```python
from build123d import *

# Parameters (mm, degrees)
TABAN_FLAN_1_DEPTH     = 5
IZGIDEN_START          = -60
IZGIDEN_B_KME2_DEPTH   = 60
IZGIDEN_B_KME2_2_DEPTH = 60
IZIM8_R                = 4.25
KES_EKSTR_ZYON1_DEPTH  = 10
RADYUS1_R              = 20
RADYUS2_R              = 5
IZIM9_R                = 4.25
KES_EKSTR_ZYON2_DEPTH  = 19


# Read off the part's stored shape, not the designer's step: Çizgiden Bükme2
# Sheet-metal steps are written as plain solids
with BuildPart() as part:
    # Çizim1 → Taban-Flanş1 (new body)
    with BuildSketch(Plane.XY):
        Polygon((0, 0), (-80, 0), (-120, -60), (-120, -115), (-50, -115), (-50, -60), (0, -60), align=None)
    extrude(amount=-TABAN_FLAN_1_DEPTH)

    # Çizgiden Bükme2 outline → Çizgiden Bükme2 (cut)
    with BuildSketch(Plane(origin=(0, 0, 0), x_dir=(1, 0, 0), z_dir=(0, 1, 0)).offset(IZGIDEN_START)):
        with BuildLine():
            Line((0, 5), (-31.042830313, 5))
            ThreePointArc((-31.042830313, 5), (-34.361671571, 1.351470729), (-39.105088062, 0))
            Line((-39.105088062, 0), (0, 0))
            Line((0, 0), (0, 5))
        make_face()
    extrude(amount=IZGIDEN_B_KME2_DEPTH, mode=Mode.SUBTRACT)

    # izgiden B_kme2 2 outline → izgiden B_kme2 2 (add)
    with BuildSketch(Plane(origin=(0, 0, 0), x_dir=(1, 0, 0), z_dir=(0, 1, 0)).offset(IZGIDEN_START)):
        with BuildLine():
            Line((-30.105088062, 37.894911938), (-35.105088062, 37.894911938))
            Line((-35.105088062, 37.894911938), (-35.105088062, 9))
            ThreePointArc((-35.105088062, 9), (-36.276660937, 6.171572875), (-39.105088062, 5))
            Line((-39.105088062, 5), (-31.042830313, 5))
            ThreePointArc((-31.042830313, 5), (-30.342659182, 6.945775053), (-30.105088062, 9))
            Line((-30.105088062, 9), (-30.105088062, 37.894911938))
        make_face()
    extrude(amount=IZGIDEN_B_KME2_2_DEPTH)

    # Çizim8 → Kes-Ekstrüzyon1 (cut)
    with BuildSketch(Plane.XY):
        with Locations((-70, -90)):
            Circle(IZIM8_R)
        with Locations((-95, -90)):
            Circle(IZIM8_R)
    extrude(amount=-KES_EKSTR_ZYON1_DEPTH, mode=Mode.SUBTRACT)

    # Radyus1
    radyus1_edges = [part.edges().sort_by_distance(p)[0] for p in [
        (-120, -60, -2.5),
        (-80, 0, -2.5),
    ]]
    fillet(radyus1_edges, radius=RADYUS1_R)

    # Radyus2
    radyus2_edges = [part.edges().sort_by_distance(p)[0] for p in [
        (-32.605088062, -60, -37.894911938),
        (-32.605088062, 0, -37.894911938),
        (-120, -115, -2.5),
        (-50, -115, -2.5),
        (-50, -60, -2.5),
    ]]
    fillet(radyus2_edges, radius=RADYUS2_R)

    # Çizim9 → Kes-Ekstrüzyon2 (cut)
    with BuildSketch(Plane.ZY.offset(35.105088062)):
        with Locations((-27.894911938, -15)):
            Circle(IZIM9_R)
        with Locations((-27.894911938, -45)):
            Circle(IZIM9_R)
    extrude(amount=-KES_EKSTR_ZYON2_DEPTH, mode=Mode.SUBTRACT)


solid = part.part
```
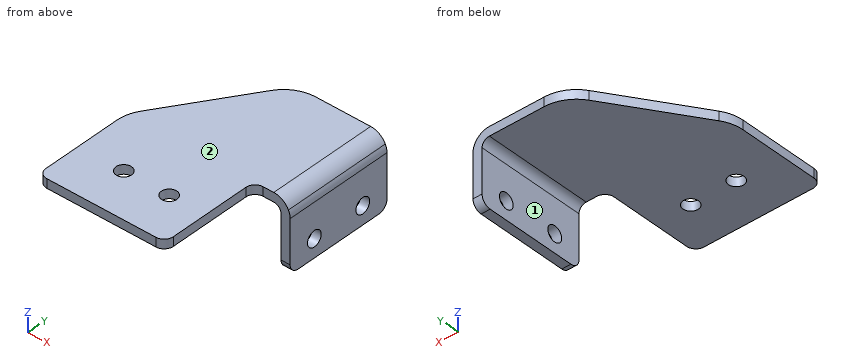
The model under review builds one solid part; all positions refer to its coordinate system, in mm. Face numbers are marked on the shaded views. A direction names the side the tool comes from. Give positions to 0.01 mm unless a question says otherwise; leave off trailing zeros. Write each loop counter-clockwise with the first axis right and the second up, starting at its lowest first coordinate (ties: lowest second). Pieces come first, ordered by that corner, then holes. Notation, with made-up numbers: (-28.75, 44.25) - (-24.75, 44.25) arc R24 cw to (-24.75, 75.25) - close; hole circle Ø3 at (89.5, 79). An arc over 180 degrees is marked (long way). Answer in a Markdown table with one row per item. Add a question column.
1. We need section B-B on y = -90. Write out the cut boundary in (x, z).
2. We need section A-A on y = -15. Write out the cut boundary in (x, z).
3. We need section C-C on x = -95. Write out the cut boundary in (y, z).
4. Insertion check: P1, Ø13.5, axis at x = -95, y = -90, coming from the -Z side; P2, Ø10, axis at x = -66, y = -47, coming from the +Z side; P3, Ø16.5, axis at x = -34.5, z = -15.5, coming from the -Y side; P4, Ø1.5, axis at y = -77.5, z = -2, coming from the +X side. Each pin has a flat end and moves straight along its axis. Give the tip position at first contact, or say it passes through.
5. Wall thickness on line 1 along Y through (x, z) = (-70, -1.85); line 2 along Z through (x, y) = (-89.5, -90.5); line 3 along Y through (x, z) = (-67, -1.5): over which ranges is each line inside the solid? List them lowest first. Write a range as [from, to].
6. We need section D-D on z = -27. Write out the cut boundary in (x, y), then the cut area to 3 significant figures.
7. Tool access review of the marked faces 1 and 2: name each direction out of +Z, -Z, +X, -X, +Y, -Y from which nothing blocks a thin tool from reaching the whole face with its end or side.
Ans:
| question | item | result |
|---|---|---|
| 1 | outline | (-120, -5) - (-99.25, -5) - (-99.25, 0) - (-120, 0) - close; (-90.75, -5) - (-74.25, -5) - (-74.25, 0) - (-90.75, 0) - close; (-65.75, -5) - (-50, -5) - (-50, 0) - (-65.75, 0) - close |
| 2 | outline | (-90, -5) - (-39.11, -5) arc R4 cw to (-35.11, -9) - (-35.11, -23.64) - (-30.11, -23.64) - (-30.11, -9) arc R9 ccw to (-39.11, 0) - (-90, 0) - close; (-35.11, -37.89) - (-30.11, -37.89) - (-30.11, -32.14) - (-35.11, -32.14) - close |
| 3 | outline | (-115, -5) - (-94.25, -5) - (-94.25, 0) - (-115, 0) - close; (-85.75, -5) - (-22.5, -5) - (-22.5, 0) - (-85.75, 0) - close |
| 4 | P1 | stops at z = -5 |
| 4 | P2 | stops at z = 0 |
| 4 | P3 | stops at y = -60 |
| 4 | P4 | stops at x = -50 |
| 5 | line 1 | y = [-115, -94.25], [-85.75, -0.01] |
| 5 | line 2 | z = [-5, 0] |
| 5 | line 3 | y = [-115, -93.01], [-86.99, 0] |
| 6 | outline | (-35.11, -60) - (-30.11, -60) - (-30.11, -49.15) - (-35.11, -49.15) - close; (-35.11, -40.85) - (-30.11, -40.85) - (-30.11, -19.15) - (-35.11, -19.15) - close; (-35.11, -10.85) - (-30.11, -10.85) - (-30.11, 0) - (-35.11, 0) - close |
| 6 | area | 217 mm^2 |
| 7 | face 1 | -Z, -X, +Y, -Y |
| 7 | face 2 | +Z, +X, -X, +Y, -Y |
